Build history of the part. All positions in model axes, mm. Face numbers are marked on the shaded views. Give positions to 0.01 mm unless a question says otherwise; leave off trailing zeros. Write each loop counter-clockwise with the first axis right and the second up, starting at its lowest first coordinate (ties: lowest second). Pieces come first, ordered by that corner, then holes. Notation, with made-up numbers: (33.5, -12) -> (72.5, -12) arc R8 ccw to (72.5, -8) -> close; hole circle Ø1 at (10.25, -2). An arc over 180 degrees is marked (long way). One line per question, with ' | ' between items. Start each with the question number.
(1) Band-saw the part on B-B, the plane x = -12.5. Give the cut face in (y, z).
(2) Pin check, flat tips, straight feed: P1, Ø4.5, axis at x = -12.5, z = -12.5, coming from the -Y side; P2, Ø3, axis at x = 12.5, z = -12.5, coming from the +Y side. Stop position of each tip, or through.
(3) Band-saw the part on C-C, the plane x = 0. Give the cut face in (y, z).
(4) Band-saw the part on D-D, the plane y = 1.3. Give the cut face in (x, z), and give its area (3 significant figures).
(5) Drill centre lines: probe 1 along X at (y, z) = (2.6, 12.5); probe 2 along X at (y, z) = (1.75, 11). Where is each one in solid material? Low to high. Write a range as from..to.
(6) Pull direction X, two halves, no side cores. Call the marked faces 1 and 2: released by +X, released by -X, zero draft, split by the parting line, or undercut.
(7) Band-saw the part on A-A, the plane z = 0. Give the cut face in (x, y).
from build123d import *

# Parameters (mm, degrees)
SKETCH1_W                  = 31.5
SKETCH1_H                  = 31.5
BOSS_EXTRUDE1_DEPTH        = 4
F_3_5_3_5_DIAMETER_HOLE1_D = 3.5
F_1_4_28_TAPPED_HOLE1_D    = 5.4102


with BuildPart() as part:
    # Sketch1 → Boss-Extrude1 (new body)
    with BuildSketch(Plane(origin=(0, 0, 0), x_dir=(1, 0, 0), z_dir=(0, 1, 0))):
        Rectangle(SKETCH1_W, SKETCH1_H)
    extrude(amount=BOSS_EXTRUDE1_DEPTH)

    # Ø3.5 (3.5) Diameter Hole1 (through all)
    with Locations(Plane(origin=(0, 4, 0), x_dir=(1, 0, 0), z_dir=(0, 1, 0))):
        with Locations((-12.5, 12.5), (12.5, 12.5), (12.5, -12.5), (-12.5, -12.5)):
            Hole(F_3_5_3_5_DIAMETER_HOLE1_D / 2)

    # 1/4-28 Tapped Hole1 (through all)
    with Locations(Plane(origin=(0, 4, 0), x_dir=(1, 0, 0), z_dir=(0, 1, 0))):
        with Locations((0, 0)):
            Hole(F_1_4_28_TAPPED_HOLE1_D / 2)


solid = part.part
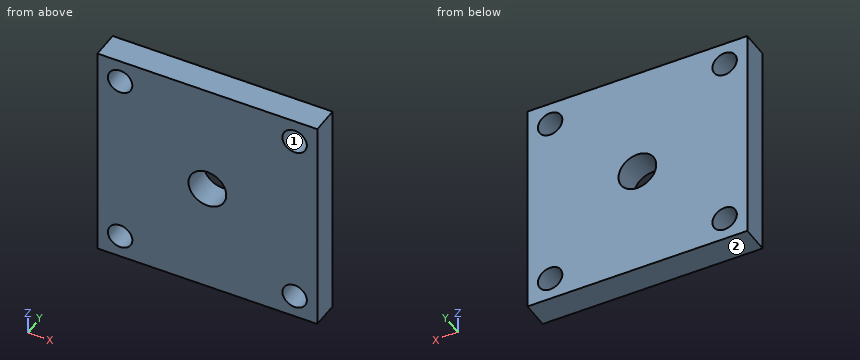
Results:
1) outline: (0, -15.75) -> (4, -15.75) -> (4, -14.25) -> (0, -14.25) -> close; (0, -10.75) -> (4, -10.75) -> (4, 10.75) -> (0, 10.75) -> close; (0, 14.25) -> (4, 14.25) -> (4, 15.75) -> (0, 15.75) -> close
2) P1: stops at y = 0 | P2: passes through
3) outline: (0, -15.75) -> (4, -15.75) -> (4, -2.71) -> (0, -2.71) -> close; (0, 2.71) -> (4, 2.71) -> (4, 15.75) -> (0, 15.75) -> close
4) outline: (-15.75, -15.75) -> (15.75, -15.75) -> (15.75, 15.75) -> (-15.75, 15.75) -> close; hole circle Ø3.5 at (-12.5, -12.5); hole circle Ø3.5 at (-12.5, 12.5); hole circle Ø5.41 at (0, 0); hole circle Ø3.5 at (12.5, -12.5); hole circle Ø3.5 at (12.5, 12.5) | area: 931 mm²
5) probe 1: x = -15.75..-14.25, -10.75..10.75, 14.25..15.75 | probe 2: x = -15.75..-13.4, -11.6..11.6, 13.4..15.75
6) face 1: undercut | face 2: zero draft
7) outline: (-15.75, 0) -> (-2.71, 0) -> (-2.71, 4) -> (-15.75, 4) -> close; (2.71, 0) -> (15.75, 0) -> (15.75, 4) -> (2.71, 4) -> close
